Input: part model. Units: mm. Frame: model coordinates. Face numbers are marked on the shaded views. A direction names the side the tool comes from. Give positions to 0.01 mm unless a question says otherwise; leave off trailing zeros. Loops run counter-clockwise (first coordinate to the right, second up) from the corner with the lowest first, then second, coordinate; pieces in that order, holes last. Notation, with made-up numbers: M 17,34.5 L 53,34.5 A36 ccw 53,73.5 Z; hole C 41.5,43.5 d11. An arc over 180 degrees is marked long. Answer as a JSON object with one key per item and string values. Group by question number.
1) Section query A-A on y = -221. Count the separate pieces of the cut face and the enclosed holes in it, plus the area to 3 significant figures.
2) Access query for the marked faces 4 and 5. Directions: +Z, -Z, +X, -X, +Y, -Y. A direction counts if a zero-diameter tool reaches every point of the face in a straight line with its end or side. Return the directions, or none.
3) Draft query along Z for the marked faces 1, 2 and 3. Return one class per face: +Z half, -Z half, draft (parallel to the pull), parting line (faces both ways), or undercut.
4) First-contact query: P1, Ø1, axis at x = -641.5, z = -173.5, coming from the -Y side. Flat tip, straight axial feed; report the tip coordinate or a pass-through.
5) Ray query, L1, parallel to Z at x = 711, y = -236; L2, parallel to Y at x = -617, z = -253.5. Return the intervals inside material, ascending.
6) Section query B-B on x = -104.5. Return loops of the section in (y, z), plus the area to 4 significant figures.
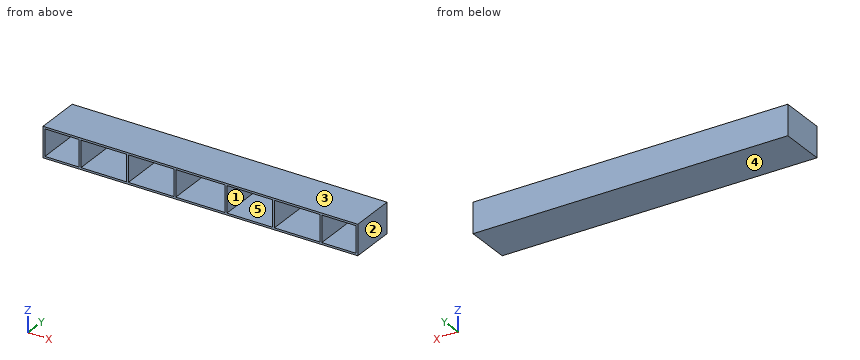
from build123d import *

# Parameters (mm, degrees)
F0_W     = 2108.2
F0_H     = 203.2
F1_DEPTH = 304.8
F2_T     = -12.7
F3_W     = 12.7
F3_H     = 177.8
F4_DEPTH = 292.1


with BuildPart() as f1:
    # F0 (on Front) → F1 (new body)
    with BuildSketch(Plane.XZ):
        with Locations((2.945067, -238.425421)):
            Rectangle(F0_W, F0_H)
    extrude(amount=F1_DEPTH)

    # F2
    f2_openings = [f1.faces().sort_by_distance(p)[0] for p in [
        (2.945067, -304.8, -238.425421),
    ]]
    offset(amount=F2_T, openings=f2_openings)

    # F3 (on face) → F4 (join)
    with BuildSketch(Plane.XZ.offset(12.7)):
        with Locations((-803.504933, -238.425421)):
            Rectangle(F3_W, F3_H)
        with Locations((-486.004933, -238.425421)):
            Rectangle(F3_W, F3_H)
        with Locations((-168.504933, -238.425421)):
            Rectangle(F3_W, F3_H)
        with Locations((174.395067, -238.425421)):
            Rectangle(F3_W, F3_H)
        with Locations((491.895067, -238.425421)):
            Rectangle(F3_W, F3_H)
        with Locations((809.395067, -238.425421)):
            Rectangle(F3_W, F3_H)
    extrude(amount=F4_DEPTH)


solid = f1.part
Output:
{
 "1": {"separate pieces": "1", "enclosed holes": "7", "area": "71,600 mm^2"},
 "2": {"face 4": "-Z, +X, -X, +Y, -Y", "face 5": "-Y"},
 "3": {"face 1": "undercut", "face 2": "draft", "face 3": "+Z half"},
 "4": {"P1": "stops at y = -12.7"},
 "5": {"L1": "z = -340.03 to -327.33, -149.53 to -136.83", "L2": "y = -12.7 to 0"},
 "6": {"outline": "M -304.8,-340.03 L 0,-340.03 L 0,-136.83 L -304.8,-136.83 L -304.8,-149.53 L -12.7,-149.53 L -12.7,-327.33 L -304.8,-327.33 Z", "area": "10,000 mm^2"}
}
